Geometry: final body of the model. Coordinates: model frame, mm. Face numbers are marked on the shaded views. Give positions to 0.01 mm unless a question says otherwise; leave off trailing zeros. Write each loop counter-clockwise with the first axis right and the second up, starting at its lowest first coordinate (ties: lowest second). Pieces come first, ordered by that corner, then holes.
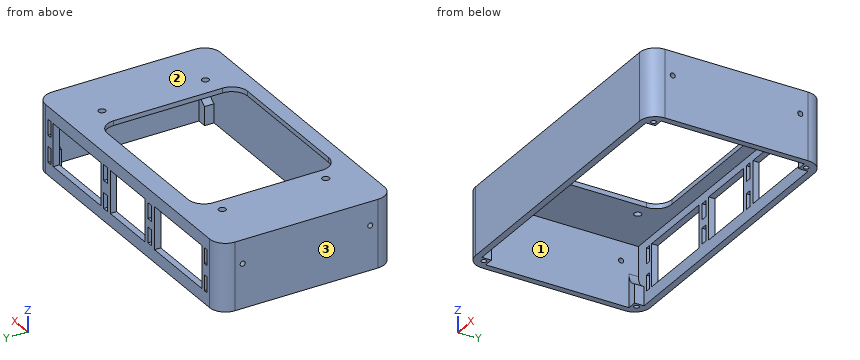
from build123d import *

# Parameters (mm, degrees)
SKETCH1_R           = 2.25
BOSS_EXTRUDE1_DEPTH = 3
BOSS_EXTRUDE3_DEPTH = 40
SKETCH4_W           = 6
SKETCH4_H           = 6
SKETCH4_R           = 1.6
BOSS_EXTRUDE4_DEPTH = 10
SKETCH5_W           = 6
SKETCH5_H           = 6
BOSS_EXTRUDE5_DEPTH = 2
FILLET3_R           = 10
SKETCH6_W           = 50
SKETCH6_H           = 27
SKETCH6_W_2         = 36.5
CUT_EXTRUDE1_DEPTH  = 5
SKETCH8_W           = 4
SKETCH8_H           = 10
SKETCH8_W_2         = 3
CUT_EXTRUDE2_DEPTH  = 5
SKETCH9_R           = 1.6
CUT_EXTRUDE3_DEPTH  = 252.455517463


with BuildPart() as part:
    # Sketch1 → Boss-Extrude1 (new body)
    with BuildSketch(Plane.XY):
        with BuildLine():
            Line((-13.577349449, 155.963544659), (-186.077349449, 155.963544659))
            ThreePointArc((-186.077349449, 155.963544659), (-193.148417261, 153.034612471), (-196.077349449, 145.963544659))
            Line((-196.077349449, 145.963544659), (-196.077349449, 54.963544659))
            ThreePointArc((-196.077349449, 54.963544659), (-193.148417261, 47.892476847), (-186.077349449, 44.963544659))
            Line((-186.077349449, 44.963544659), (-13.577349449, 44.963544659))
            ThreePointArc((-13.577349449, 44.963544659), (-6.506281637, 47.892476847), (-3.577349449, 54.963544659))
            Line((-3.577349449, 54.963544659), (-3.577349449, 145.963544659))
            ThreePointArc((-3.577349449, 145.963544659), (-6.506281637, 153.034612471), (-13.577349449, 155.963544659))
        make_face()
        with Locations((-35.292149682, 133.289732278)):
            Circle(SKETCH1_R, mode=Mode.SUBTRACT)
        with Locations((-35.297563809, 67.599891559)):
            Circle(SKETCH1_R, mode=Mode.SUBTRACT)
        with Locations((-161.808024727, 67.580045294)):
            Circle(SKETCH1_R, mode=Mode.SUBTRACT)
        with Locations((-161.808423577, 133.28851775)):
            Circle(SKETCH1_R, mode=Mode.SUBTRACT)
        with BuildLine():
            Line((-57.8741303, 143.534465984), (-142.973432949, 143.534465984))
            ThreePointArc((-142.973432949, 143.534465984), (-150.044500761, 140.605533796), (-152.973432949, 133.534465984))
            Line((-152.973432949, 133.534465984), (-152.973432949, 64.356832554))
            ThreePointArc((-152.973432949, 64.356832554), (-150.044500761, 57.285764742), (-142.973432949, 54.356832554))
            Line((-142.973432949, 54.356832554), (-57.8741303, 54.356832554))
            ThreePointArc((-57.8741303, 54.356832554), (-50.803062488, 57.285764742), (-47.8741303, 64.356832554))
            Line((-47.8741303, 64.356832554), (-47.8741303, 133.534465984))
            ThreePointArc((-47.8741303, 133.534465984), (-50.803062488, 140.605533796), (-57.8741303, 143.534465984))
        make_face(mode=Mode.SUBTRACT)
    extrude(amount=-BOSS_EXTRUDE1_DEPTH)

    # Sketch3 → Boss-Extrude3 (add)
    with BuildSketch(Plane(origin=(0, 0, -3), x_dir=(-1, 0, 0), z_dir=(0, 0, -1))):
        with BuildLine():
            Line((3.577349449, 145.963544659), (3.577349449, 54.963544659))
            ThreePointArc((3.577349449, 54.963544659), (6.506281637, 47.892476847), (13.577349449, 44.963544659))
            Line((13.577349449, 44.963544659), (99.827349449, 44.963544659))
            Line((99.827349449, 44.963544659), (186.077349449, 44.963544659))
            ThreePointArc((186.077349449, 44.963544659), (193.148417261, 47.892476847), (196.077349449, 54.963544659))
            Line((196.077349449, 54.963544659), (196.077349449, 145.963544659))
            ThreePointArc((196.077349449, 145.963544659), (193.148417261, 153.034612471), (186.077349449, 155.963544659))
            Line((186.077349449, 155.963544659), (99.827349449, 155.963544659))
            Line((99.827349449, 155.963544659), (13.577349449, 155.963544659))
            ThreePointArc((13.577349449, 155.963544659), (6.506281637, 153.034612471), (3.577349449, 145.963544659))
        make_face()
        Polygon((7.577349449, 151.963544659), (7.577349449, 48.963544659), (99.827349449, 48.963544659), (192.077349449, 48.963544659), (192.077349449, 151.963544659), (99.827349449, 151.963544659), align=None, mode=Mode.SUBTRACT)
    extrude(amount=BOSS_EXTRUDE3_DEPTH)

    # Sketch4 → Boss-Extrude4 (add)
    # profile 1 of 4: a face of its own
    with BuildSketch(Plane(origin=(0, 0, -43), x_dir=(-1, 0, 0), z_dir=(0, 0, -1))):
        with Locations((10.577349449, 148.963544659)):
            Rectangle(SKETCH4_W, SKETCH4_H)
        with Locations((10.577349449, 148.963544659)):
            Circle(SKETCH4_R, mode=Mode.SUBTRACT)
    # profile 2 of 4: a face of its own
    with BuildSketch(Plane(origin=(0, 0, -43), x_dir=(-1, 0, 0), z_dir=(0, 0, -1))):
        with Locations((189.077349449, 148.963544659)):
            Rectangle(SKETCH4_W, SKETCH4_H)
        with Locations(Location((189.077349449, 148.963544659, 0), (0, 0, 180))):
            Circle(SKETCH4_R, mode=Mode.SUBTRACT)
    # profile 3 of 4: a face of its own
    with BuildSketch(Plane(origin=(0, 0, -43), x_dir=(-1, 0, 0), z_dir=(0, 0, -1))):
        with Locations((189.077349449, 51.963544659)):
            Rectangle(SKETCH4_W, SKETCH4_H)
        with Locations(Location((189.077349449, 51.963544659, 0), (0, 0, 180))):
            Circle(SKETCH4_R, mode=Mode.SUBTRACT)
    # profile 4 of 4: a face of its own
    with BuildSketch(Plane(origin=(0, 0, -43), x_dir=(-1, 0, 0), z_dir=(0, 0, -1))):
        with Locations((10.577349449, 51.963544659)):
            Rectangle(SKETCH4_W, SKETCH4_H)
        with Locations((10.577349449, 51.963544659)):
            Circle(SKETCH4_R, mode=Mode.SUBTRACT)
    extrude(amount=-BOSS_EXTRUDE4_DEPTH)

    # Sketch5 → Boss-Extrude5 (add)
    with BuildSketch(Plane.XY.offset(-33)):
        with Locations((-189.077349449, 148.963544659)):
            Rectangle(SKETCH5_W, SKETCH5_H)
        with Locations((-189.077349449, 51.963544659)):
            Rectangle(SKETCH5_W, SKETCH5_H)
        with Locations((-10.577349449, 51.963544659)):
            Rectangle(SKETCH5_W, SKETCH5_H)
        with Locations((-10.577349449, 148.963544659)):
            Rectangle(SKETCH5_W, SKETCH5_H)
    extrude(amount=BOSS_EXTRUDE5_DEPTH)

    # Fillet3
    # the kernel refuses this fillet: 10 mm, written as the material it adds along each edge
    with BuildSketch(Plane(origin=(-192.077349449, 145.963544659, -31), x_dir=(1, 0, 0), z_dir=(0, 1, 0)), Plane(origin=(-7.577349449, 151.963544659, -31), x_dir=(-1, 0, 0), z_dir=(0, -1, 0))) as fillet3_piece_1:
        with BuildLine():
            CenterArc((10, -9.16515139), FILLET3_R, 113.578178478, 66.421821522)
            Line((0, -9.16515139), (-0.2, -9.16515139))
            Line((-0.2, -9.16515139), (-0.2, 0))
            Line((-0.2, 0), (0, 0.2))
            ThreePointArc((0, 0.2), (3, 0.2), (5.92, 0.183303028))
            Line((5.92, 0.183303028), (6, 0))
        make_face()
    extrude(amount=6)
    with BuildSketch(Plane(origin=(-192.077349449, 48.963544659, -31), x_dir=(0, 0, 1), z_dir=(0, 1, 0))) as fillet3_piece_2:
        with BuildLine():
            CenterArc((9.16515139, 10), FILLET3_R, 203.578178478, 66.421821522)
            Line((0, 6), (-0.183303028, 5.92))
            ThreePointArc((-0.183303028, 5.92), (-0.2, 3), (-0.2, 0))
            Line((-0.2, 0), (0, -0.2))
            Line((0, -0.2), (9.16515139, -0.2))
            Line((9.16515139, -0.2), (9.16515139, 0))
        make_face()
    extrude(amount=6)
    with BuildSketch(Plane(origin=(-7.577349449, 48.963544659, -31), x_dir=(-1, 0, 0), z_dir=(0, 1, 0))) as fillet3_piece_3:
        with BuildLine():
            CenterArc((10, 9.16515139), FILLET3_R, 180, 66.421821522)
            Line((0, 9.16515139), (-0.2, 9.16515139))
            Line((-0.2, 9.16515139), (-0.2, 0))
            Line((-0.2, 0), (0, -0.2))
            ThreePointArc((0, -0.2), (3, -0.2), (5.92, -0.183303028))
            Line((5.92, -0.183303028), (6, 0))
        make_face()
    extrude(amount=6)

    # Sketch6 → Cut-Extrude1 (cut)
    with BuildSketch(Plane(origin=(0, 155.963544659, 0), x_dir=(1, 0, 0), z_dir=(0, 1, 0))):
        with Locations((-153.077349449, 21.5)):
            Rectangle(SKETCH6_W, SKETCH6_H)
        with Locations((-99.827349449, 21.5)):
            Rectangle(SKETCH6_W_2, SKETCH6_H)
        with Locations((-46.577349449, 21.5)):
            Rectangle(SKETCH6_W, SKETCH6_H)
    extrude(amount=-CUT_EXTRUDE1_DEPTH, mode=Mode.SUBTRACT)

    # Sketch8 → Cut-Extrude2 (cut)
    with BuildSketch(Plane(origin=(0, 155.963544659, 0), x_dir=(1, 0, 0), z_dir=(0, 1, 0))):
        with Locations((-123.077349449, 13.876287988)):
            Rectangle(SKETCH8_W, SKETCH8_H)
        with Locations((-76.577349449, 12.724006881)):
            Rectangle(SKETCH8_W, SKETCH8_H)
        with Locations((-76.577349449, 30.275993119)):
            Rectangle(SKETCH8_W, SKETCH8_H)
        with Locations((-123.077349449, 29.123712012)):
            Rectangle(SKETCH8_W, SKETCH8_H)
        with Locations((-17.577349449, 13)):
            Rectangle(SKETCH8_W_2, SKETCH8_H)
        with Locations((-182.077349449, 13)):
            Rectangle(SKETCH8_W_2, SKETCH8_H)
        with Locations((-17.577349449, 30)):
            Rectangle(SKETCH8_W_2, SKETCH8_H)
        with Locations((-182.077349449, 30)):
            Rectangle(SKETCH8_W_2, SKETCH8_H)
    extrude(amount=-CUT_EXTRUDE2_DEPTH, mode=Mode.SUBTRACT)

    # Sketch9 → Cut-Extrude3 (cut, through all)
    with BuildSketch(Plane(origin=(-3.577349449, 0, 0), x_dir=(0, 0, -1), z_dir=(1, 0, 0))):
        with Locations(Location((15, 140.963544659, 0), (0, 0, 90))):
            Circle(SKETCH9_R)
        with Locations(Location((15, 59.963544659, 0), (0, 0, 90))):
            Circle(SKETCH9_R)
    extrude(amount=-CUT_EXTRUDE3_DEPTH, mode=Mode.SUBTRACT)


solid = part.part
Q1. Section C-C on y = 115. Output: boundary loops of the cut face in (x, z).
Filled sheet:
outline: (-196.08, -43) - (-192.08, -43) - (-192.08, -3) - (-152.97, -3) - (-152.97, 0) - (-196.08, 0) - close; (-47.87, -3) - (-7.58, -3) - (-7.58, -43) - (-3.58, -43) - (-3.58, 0) - (-47.87, 0) - close
Q2. Ray query, line 1 along X through (y, z) = (88, -27.5); line 2 along Y through (x, z) = (-68.5, -40); line 3 along Z through (x, y) = (-174, 50). Return the intervals inside material, ascending.
Filled sheet:
line 1: x = -196.08 to -192.08, -7.58 to -3.58
line 2: y = 44.96 to 48.96, 151.96 to 155.96
line 3: z = -3 to 0
Q3. Pull-direction query (X, two-part tool) for the marked faces 1, 2 and 3; classes: released by +X, released by -X, zero draft, split by the parting line, or undercut.
Filled sheet:
face 1: undercut
face 2: zero draft
face 3: released by -X
Q4. Section A-A on x = -45.5. Output: boundary loops of the cut face in (y, z), plus the area to 3 significant figures.
Filled sheet:
outline: (44.96, -43) - (48.96, -43) - (48.96, -3) - (151.96, -3) - (151.96, -8) - (155.96, -8) - (155.96, 0) - (44.96, 0) - close; (151.96, -43) - (155.96, -43) - (155.96, -35) - (151.96, -35) - close
area: 545 mm2
Q5. Section D-D on z = -28.5. Count the separate pieces of the cut face and the enclosed holes in it, plus the area to 3 significant figures.
Filled sheet:
separate pieces: 7
enclosed holes: 0
area: 1,740 mm2
Q6. Section B-B on x = -138. Output: boundary loops of the cut face in (y, z), plus the area to 3 significant figures.
Filled sheet:
outline: (44.96, -43) - (48.96, -43) - (48.96, -3) - (54.36, -3) - (54.36, 0) - (44.96, 0) - close; (143.53, -3) - (151.96, -3) - (151.96, -8) - (155.96, -8) - (155.96, 0) - (143.53, 0) - close; (151.96, -43) - (155.96, -43) - (155.96, -35) - (151.96, -35) - close
area: 277 mm2
Q7. Pin query (flat end, axial travel): P1, Ø12, axis at x = -123.5, y = 60, coming from the -Z side; P2, Ø4.5, axis at y = 153, z = -28.5, coming from the +X side; P3, Ø5, axis at y = 51.5, z = -35, coming from the -X side. Return the tip coordinate at first contact, or that it passes through.
Filled sheet:
P1: stops at z = -3
P2: stops at x = -4.8
P3: stops at x = -196.03
